from build123d import *

# Parameters (mm, degrees)
SKETCH1_W           = 51
SKETCH1_H           = 51
BOSS_EXTRUDE1_DEPTH = 2.8
SKETCH2_R           = 11
SKETCH2_R_2         = 1.7
CUT_EXTRUDE1_DEPTH  = 3.8


with BuildPart() as part:
    # Sketch1 → Boss-Extrude1 (new body)
    with BuildSketch(Plane.XY):
        Rectangle(SKETCH1_W, SKETCH1_H)
    extrude(amount=BOSS_EXTRUDE1_DEPTH)

    # Sketch2 → Cut-Extrude1 (cut, through all)
    with BuildSketch(Plane(origin=(0, 0, 0), x_dir=(-1, 0, 0), z_dir=(0, 0, -1))):
        with Locations((0, 4.5)):
            Circle(SKETCH2_R)
        with Locations((-15.5, 20)):
            Circle(SKETCH2_R_2)
        with Locations((15.5, 20)):
            Circle(SKETCH2_R_2)
        with Locations((15.5, -11)):
            Circle(SKETCH2_R_2)
        with Locations((-15.5, -11)):
            Circle(SKETCH2_R_2)
        with Locations((-9.899494937, 14.399494937)):
            Circle(SKETCH2_R_2)
        with Locations((9.899494937, 14.399494937)):
            Circle(SKETCH2_R_2)
        with Locations((9.899494937, -5.399494937)):
            Circle(SKETCH2_R_2)
        with Locations((-9.899494937, -5.399494937)):
            Circle(SKETCH2_R_2)
    extrude(amount=-CUT_EXTRUDE1_DEPTH, mode=Mode.SUBTRACT)


solid = part.part
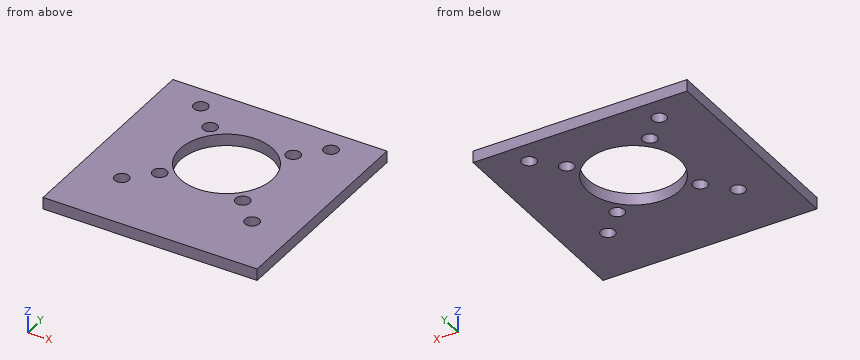
Geometry check sheet. Reference: the model listing, model coordinates, mm. Round coordinates to 2 decimals unless told otherwise and drop trailing zeros. Loops run counter-clockwise (first coordinate to the right, second up) from the corner with the lowest first, then second, coordinate; pieces in that order, holes last. Notation, with made-up numbers: (86, 28.25) -> (128, 28.25) arc R19 cw to (128, 64.25) -> close; hole circle Ø6 at (-26.5, -31). An arc over 180 degrees is marked (long way). Answer as a JSON object with one key per item and string values. Group by question number.
Item 1: Cross-section at D-D, the plane y = 9. Record the cut outline in (x, z), plus the area to 3 significant figures.
Item 2: Cross-section at A-A, the plane x = 0. Record the cut outline in (y, z), plus the area to 3 significant figures.
Item 3: Cross-section at C-C, the plane y = 20. Record the cut outline in (x, z).
Item 4: Cross-section at B-B, the plane x = 15.5. Record the cut outline in (y, z), plus the area to 3 significant figures.
Item 5: Thickness scan on line 1 along Y through (x, z) = (-15.5, 1.2); line 2 along Y through (x, z) = (-14, 0.2); line 3 along X through (y, z) = (21, 0.8). Record the ranges inside material, lowest first.
Determined:
{
 "1": {"outline": "(-25.5, 0) -> (-10.04, 0) -> (-10.04, 2.8) -> (-25.5, 2.8) -> close; (10.04, 0) -> (25.5, 0) -> (25.5, 2.8) -> (10.04, 2.8) -> close", "area": "86.6 mm²"},
 "2": {"outline": "(-25.5, 0) -> (-6.5, 0) -> (-6.5, 2.8) -> (-25.5, 2.8) -> close; (15.5, 0) -> (25.5, 0) -> (25.5, 2.8) -> (15.5, 2.8) -> close", "area": "81.2 mm²"},
 "3": {"outline": "(-25.5, 0) -> (-17.2, 0) -> (-17.2, 2.8) -> (-25.5, 2.8) -> close; (-13.8, 0) -> (13.8, 0) -> (13.8, 2.8) -> (-13.8, 2.8) -> close; (17.2, 0) -> (25.5, 0) -> (25.5, 2.8) -> (17.2, 2.8) -> close"},
 "4": {"outline": "(-25.5, 0) -> (-12.7, 0) -> (-12.7, 2.8) -> (-25.5, 2.8) -> close; (-9.3, 0) -> (18.3, 0) -> (18.3, 2.8) -> (-9.3, 2.8) -> close; (21.7, 0) -> (25.5, 0) -> (25.5, 2.8) -> (21.7, 2.8) -> close", "area": "124 mm²"},
 "5": {"line 1": "y = -25.5 to -12.7, -9.3 to 18.3, 21.7 to 25.5", "line 2": "y = -25.5 to -11.8, -10.2 to 19.2, 20.8 to 25.5", "line 3": "x = -25.5 to -16.87, -14.13 to 14.13, 16.87 to 25.5"}
}
